Read the model definition and answer for the solid it produces. Units are mm, in the model's axes. A direction names the side the tool comes from. Coordinates: 2 decimals unless noted, no trailing zeros. Loops run counter-clockwise (first coordinate to the right, second up) from the corner with the lowest first, then second, coordinate; pieces in that order, holes last. Notation, with made-up numbers: (19.25, -17) -> (41.25, -17) arc R15 ccw to (41.25, -12) -> close; hole circle Ø1 at (63, 14). An arc over 180 degrees is marked (long way). Answer as a JSON object with one key per item and string values. Group by question number.
Q1. For faces 1 (the flat face through (-36, 19, 8)), 2 (the flat face through (-23, 0, -9)), 3 (the flat face through (11.661, 0.378, 27.084)), 4 (the flat face through (36, -19, 8)), 5 (the flat face through (-33, 0, 33)), determine the directions among +Z, -Z, +X, -X, +Y, -Y from which every point of the face is accessible in a straight line to the end or side of a thin tool.
Q2. The part is cut by section A-A on y = -11. Write down the section's boundary in (x, z), and give its area (3 significant figures).
Q3. The part is cut by section B-B on x = -40.5. Write down the section's boundary in (y, z).
Q4. Determine the mould class of faces 6 (the flat face through (40.367, 23.056, -2.322)), 7 (the flat face through (-11.339, 0.378, 26.916)), 8 (the flat face through (36, 19, 8)) for opening direction X: released by +X, released by -X, zero draft, split by the parting line, or undercut.
Q5. Each of these flat-tipped pins is pushed along its axis until it touches: P1, Ø3, axis at x = 1, y = 11.5, coming from the +Z side; P2, Ø14, axis at x = -40.5, y = 0, coming from the -Z side; P3, Ø1.5, axis at y = -3.5, z = -3.5, coming from the +X side. Where does it stop, or does it pass through?
Q6. The part is cut by section D-D on z = -19. Write down the section's boundary in (x, y), and give its area (3 significant figures).
Q7. The part is cut by section C-C on z = 24.5. Write down the section's boundary in (x, y).
Q8. Straight lines are drawn through the part: line 1 along X through (y, z) = (-13, 0); line 2 along Y through (x, z) = (-34.5, -7.5); line 3 along X through (y, z) = (-16, -7.5). For each, find the intervals that lie inside material, in ascending order. Write a range as [from, to].
from build123d import *

# Parameters (mm, degrees)
SKETCH_1_R          = 7
EXTRUDE_1_DEPTH     = 27
SKETCH_2_W          = 19
SKETCH_2_H          = 38
SKETCH_2_R          = 6
CUT_EXTRUDE_1_DEPTH = 46
SKETCH_2_2_R        = 6
CUT_EXTRUDE_2_DEPTH = 82.197290595


with BuildPart() as part:
    # 草图1 → 凸台-拉伸1 (new, symmetric)
    with BuildSketch(Plane(origin=(0, 0, 0), x_dir=(1, 0, 0), z_dir=(0, 1, 0))):
        with BuildLine():
            Line((15, 0), (15, -7))
            Line((15, -7), (23, -7))
            Line((23, -7), (23, 25))
            Line((23, 25), (31, 25))
            Line((31, 25), (50, -21))
            Line((50, -21), (50, -33))
            Line((50, -33), (23, -33))
            Line((23, -33), (0, -21))
            Line((0, -21), (-23, -33))
            Line((-23, -33), (-50, -33))
            Line((-50, -33), (-50, -21))
            Line((-50, -21), (-31, 25))
            Line((-31, 25), (-23, 25))
            Line((-23, 25), (-23, -7))
            Line((-23, -7), (-15, -7))
            Line((-15, -7), (-15, 0))
            ThreePointArc((-15, 0), (0, 15), (15, 0))
        make_face()
        with Locations(Location((0, 0, 0), (0, 0, 270))):
            Circle(SKETCH_1_R, mode=Mode.SUBTRACT)
    extrude(amount=EXTRUDE_1_DEPTH, both=True)

    # 草图2 → 切除-拉伸1 (cut)
    # profile 1 of 2: a face of its own
    with BuildSketch(Plane(origin=(0, 0, -25), x_dir=(-1, 0, 0), z_dir=(0, 0, -1))):
        with Locations((40.5, 0)):
            Rectangle(SKETCH_2_W, SKETCH_2_H)
        with Locations((40.5, 0)):
            Circle(SKETCH_2_R, mode=Mode.SUBTRACT)
    # profile 2 of 2: a face of its own
    with BuildSketch(Plane(origin=(0, 0, -25), x_dir=(-1, 0, 0), z_dir=(0, 0, -1))):
        with Locations((-40.5, 0)):
            Rectangle(SKETCH_2_W, SKETCH_2_H)
        with Locations((-40.5, 0)):
            Circle(SKETCH_2_R, mode=Mode.SUBTRACT)
    extrude(amount=-CUT_EXTRUDE_1_DEPTH, mode=Mode.SUBTRACT)

    # 草图2<2> → 切除-拉伸2 (cut, through all)
    with BuildSketch(Plane(origin=(0, 0, -25), x_dir=(-1, 0, 0), z_dir=(0, 0, -1))):
        with Locations((40.5, 0)):
            Circle(SKETCH_2_2_R)
        with Locations((-40.5, 0)):
            Circle(SKETCH_2_2_R)
    extrude(amount=-CUT_EXTRUDE_2_DEPTH, mode=Mode.SUBTRACT)


solid = part.part
Final values:
{
 "1": {"face 1": "-Z, -X", "face 2": "-Z, +Y, -Y", "face 3": "+Z, +Y, -Y", "face 4": "-Z, +X", "face 5": "+Z, +X, -X, +Y, -Y"},
 "2": {"outline": "(-50, 21) -> (-31, 21) -> (-31, -25) -> (-23, -25) -> (-23, 7) -> (-15, 7) -> (-15, 0) arc R15 ccw to (15, 0) -> (15, 7) -> (23, 7) -> (23, -25) -> (31, -25) -> (31, 21) -> (50, 21) -> (50, 33) -> (23, 33) -> (0, 21) -> (-23, 33) -> (-50, 33) -> close; hole circle Ø14 at (0, 0)", "area": "2,710 mm2"},
 "3": {"outline": "(-27, -2) -> (-19, -2) -> (-19, 21) -> (-6, 21) -> (-6, 33) -> (-27, 33) -> close; (6, 21) -> (19, 21) -> (19, -2) -> (27, -2) -> (27, 33) -> (6, 33) -> close"},
 "4": {"face 6": "released by +X", "face 7": "undercut", "face 8": "zero draft"},
 "5": {"P1": "stops at z = 22.3", "P2": "stops at z = 21", "P3": "stops at x = 31"},
 "6": {"outline": "(-33.48, -27) -> (-23, -27) -> (-23, 27) -> (-33.48, 27) -> (-33.48, 19) -> (-31, 19) -> (-31, -19) -> (-33.48, -19) -> close; (23, -27) -> (33.48, -27) -> (33.48, -19) -> (31, -19) -> (31, 19) -> (33.48, 19) -> (33.48, 27) -> (23, 27) -> close", "area": "943 mm2"},
 "7": {"outline": "(-50, -27) -> (-6.71, -27) -> (-6.71, 27) -> (-50, 27) -> close; (6.71, -27) -> (50, -27) -> (50, 27) -> (6.71, 27) -> close; hole circle Ø12 at (-40.5, 0); hole circle Ø12 at (40.5, 0)"},
 "8": {"line 1": "x = [-31, -23], [-15, -7], [7, 15], [23, 31]", "line 2": "y = [-27, -19], [19, 27]", "line 3": "x = [-31, -23], [-12.99, 12.99], [23, 31]"}
}
